```python
from build123d import *

# Parameters (mm, degrees)
SKETCH1_R           = 2.1
SKETCH1_R_2         = 4.25
BOSS_EXTRUDE1_DEPTH = 5


with BuildPart() as part:
    # Sketch1 → Boss-Extrude1 (new body)
    # profile 1 of 2: a face of its own
    with BuildSketch(Plane.XY):
        with BuildLine():
            Line((5.353571071, -17), (36.690694186, -12.889590884))
            ThreePointArc((36.690694186, -12.889590884), (48, 0), (36.690694186, 12.889590884))
            Line((36.690694186, 12.889590884), (5.353571071, 17))
            Line((5.353571071, 17), (-30.83030278, 17))
            ThreePointArc((-30.83030278, 17), (-37.5, 0), (-30.83030278, -17))
            Line((-30.83030278, -17), (5.353571071, -17))
        make_face()
        with Locations((-22.5, 13)):
            Circle(SKETCH1_R, mode=Mode.SUBTRACT)
        with Locations((-2.5, 13)):
            Circle(SKETCH1_R, mode=Mode.SUBTRACT)
        Circle(SKETCH1_R_2, mode=Mode.SUBTRACT)
        with Locations((-25, 0)):
            Circle(SKETCH1_R_2, mode=Mode.SUBTRACT)
        with Locations((-22.5, -13)):
            Circle(SKETCH1_R, mode=Mode.SUBTRACT)
        with Locations((-2.5, -13)):
            Circle(SKETCH1_R, mode=Mode.SUBTRACT)
        with BuildLine():
            ThreePointArc((44.5, 0), (35, 9.5), (25.5, 0))
            ThreePointArc((25.5, 0), (35, -9.5), (44.5, 0))
        make_face(mode=Mode.SUBTRACT)
    # profile 2 of 2: a face of its own
    with BuildSketch(Plane.XY):
        with BuildLine():
            ThreePointArc((25.5, 0), (35, -9.5), (44.5, 0))
            ThreePointArc((44.5, 0), (35, 9.5), (25.5, 0))
        make_face()
        with BuildLine():
            ThreePointArc((34.2, 7), (35, 6.2), (35.8, 7))
            ThreePointArc((35.8, 7), (35, 7.8), (34.2, 7))
        make_face(mode=Mode.SUBTRACT)
        with BuildLine():
            ThreePointArc((40.749747468, 4.949747468), (39.949747468, 5.749747468), (39.149747468, 4.949747468))
            ThreePointArc((39.149747468, 4.949747468), (39.949747468, 4.149747468), (40.749747468, 4.949747468))
        make_face(mode=Mode.SUBTRACT)
        with BuildLine():
            ThreePointArc((42.8, 0), (42, 0.8), (41.2, 0))
            ThreePointArc((41.2, 0), (42, -0.8), (42.8, 0))
        make_face(mode=Mode.SUBTRACT)
        with BuildLine():
            ThreePointArc((40.749747468, -4.949747468), (39.949747468, -4.149747468), (39.149747468, -4.949747468))
            ThreePointArc((39.149747468, -4.949747468), (39.949747468, -5.749747468), (40.749747468, -4.949747468))
        make_face(mode=Mode.SUBTRACT)
        with BuildLine():
            ThreePointArc((35.8, -7), (35, -6.2), (34.2, -7))
            ThreePointArc((34.2, -7), (35, -7.8), (35.8, -7))
        make_face(mode=Mode.SUBTRACT)
        with BuildLine():
            ThreePointArc((29.250252532, -4.949747468), (30.050252532, -5.749747468), (30.850252532, -4.949747468))
            ThreePointArc((30.850252532, -4.949747468), (30.050252532, -4.149747468), (29.250252532, -4.949747468))
        make_face(mode=Mode.SUBTRACT)
        with BuildLine():
            ThreePointArc((27.2, 0), (28, -0.8), (28.8, 0))
            ThreePointArc((28.8, 0), (28, 0.8), (27.2, 0))
        make_face(mode=Mode.SUBTRACT)
        with BuildLine():
            ThreePointArc((29.250252532, 4.949747468), (30.050252532, 4.149747468), (30.850252532, 4.949747468))
            ThreePointArc((30.850252532, 4.949747468), (30.050252532, 5.749747468), (29.250252532, 4.949747468))
        make_face(mode=Mode.SUBTRACT)
        with BuildLine():
            ThreePointArc((39.5, 0), (35, 4.5), (30.5, 0))
            ThreePointArc((30.5, 0), (35, -4.5), (39.5, 0))
        make_face(mode=Mode.SUBTRACT)
    extrude(amount=BOSS_EXTRUDE1_DEPTH)


solid = part.part
```
Verification items for the finished model (mm, model axes). Coordinates: 2 decimals unless noted, no trailing zeros. Order: outer loops, then holes, each group sorted by start corner. A loop starts at its lowest first (then second) coordinate and runs counter-clockwise, first axis right, second up. Notation, with made-up numbers: (-11, 3.5) -> (12, 3.5) arc R21 cw to (12, 30.5) -> close; hole circle Ø3 at (60, -34.5). An arc over 180 degrees is marked (long way). Put each result on its own line as item: value. Start each with the question number.
1) Release check for a two-part mould opening along Y. For faces 1 (the flat face through (21.241, 14.916, 2.465)), 2 (the cylindrical face through (42.63, 0.49, 2.46)), 3 (the cylindrical face through (48, 0, 2)) record: pulls with the +Y half, pulls with the -Y half, needs draft (parallel to the pull), parting line crosses it, or undercut.
2) Cross-section at C-C (z = 1.45). State how many separate pieces and enclosed holes the cut face has, plus the area to 3 significant figures.
3) Go/stop test with a flat-tipped pin: pin 1 (3 mm diameter, centred on y = 9.5, z = 1.5, fed in from +X). Record where the tip stops, or that it passes through.
4) Cross-section at B-B (y = 12). Enter the section's corners in (x, z).
5) Cross-section at A-A (x = 28). Enter the section's corners in (y, z).
6) Cross-section at D-D (y = -7). Enter the section's corners in (x, z), plus the area to 3 significant figures.
7) Material ranges on L1, parallel to Y at x = -25, z = 1.9; L2, parallel to X at y = 3, z = 2.9; L3, parallel to Y at x = -2.5, z = 1.2, recorded low to high.
Geometry check:
1. face 1: pulls with the +Y half
1. face 2: undercut
1. face 3: parting line crosses it
2. separate pieces: 1
2. enclosed holes: 15
2. area: 2,300 mm^2
3. pin 1: stops at x = 45.25
4. outline: (-34.43, 0) -> (-24.35, 0) -> (-24.35, 5) -> (-34.43, 5) -> close; (-20.65, 0) -> (-4.35, 0) -> (-4.35, 5) -> (-20.65, 5) -> close; (-0.65, 0) -> (40, 0) -> (40, 5) -> (-0.65, 5) -> close
5. outline: (-14.03, 0) -> (-0.8, 0) -> (-0.8, 5) -> (-14.03, 5) -> close; (0.8, 0) -> (14.03, 0) -> (14.03, 5) -> (0.8, 5) -> close
6. outline: (-36.5, 0) -> (34.2, 0) -> (34.2, 5) -> (-36.5, 5) -> close; (35.8, 0) -> (45.95, 0) -> (45.95, 5) -> (35.8, 5) -> close
6. area: 404 mm^2
7. L1: y = -17 to -4.25, 4.25 to 17
7. L2: x = -37.32 to -28.01, -21.99 to -3.01, 3.01 to 31.65, 38.35 to 47.65
7. L3: y = -17 to -15.1, -10.9 to -3.44, 3.44 to 10.9, 15.1 to 17
